Read the model definition and answer for the solid it produces. Units are mm, in the model's axes. A direction names the side the tool comes from. Round coordinates to 2 decimals unless told otherwise and drop trailing zeros. Write each loop counter-clockwise with the first axis right and the second up, starting at its lowest first coordinate (ties: lowest second). Pieces come first, ordered by that corner, then holes. Notation, with made-up numbers: (34, -17.5) - (61, -17.5) arc R29 cw to (61, 21.5) - close; hole circle Ø4 at (35, 57.5). An arc over 180 degrees is marked (long way). One line per item, written item: value. Start each with the question number.
(1) Find the intervals of material crossed by L1, parallel to X at y = 28, z = -6; L2, parallel to X at y = 11, z = -12; L3, parallel to Z at x = -45.5, y = 3, in increasing order.
(2) For faces 4 (the face through (-23, 4, -4)), 5 (the face through (-28.36, 17.04, -6.56)), 6 (the face through (0, 4.8, 0)), 7 (the face through (-35.24, 17.04, -5.67)), determine the directions among +Z, -Z, +X, -X, +Y, -Y from which every point of the face is accessible in a straight line to the end or side of a thin tool.
(3) The mould has two halves that part along Y. Classify faces 1 (the face through (10.2, 15, -3)), 2 (the face through (-25, 0, -4)), 3 (the face through (-31.82, 7.1, -9.68)): +Y half, -Y half, draft (parallel to the pull), parting line (faces both ways), or undercut.
(4) Flat-ended cylindrical pins translate along their axes: pin 1 Ø8 at (x, y) = (-36.5, 24) entering from +Z; pin 2 Ø8 at (x, y) = (-8, 17.5) entering from -Z; pin 3 Ø1.7 at (x, z) = (-54.74, -3.79) entering from +Y; pin 4 Ø4 at (x, y) = (-9.5, 8.5) entering from +Z. Find the tip coordinate at first contact, or state that the pin passes through.
(5) A cutting plane is placed at A-A, the plane y = 5.75. State how many separate pieces and enclosed holes the cut face has, plus the area to 3 significant figures.
(6) A cutting plane is placed at C-C, the plane x = 0. Determine the outline of the cut face in (y, z), plus the area to 3 significant figures.
from build123d import *

# Parameters (mm, degrees)
SKETCH1_W           = 30
SKETCH1_H           = 20
BOSS_EXTRUDE1_DEPTH = 30
SKETCH3_R           = 1.4
SKETCH3_R_2         = 5.2
BOSS_EXTRUDE2_DEPTH = 30
SKETCH2_W           = 20.4
SKETCH2_H           = 20.4
CUT_EXTRUDE1_DEPTH  = 79.115650631
SKETCH9_R           = 7.5
CUT_EXTRUDE5_DEPTH  = 75.606681327
SKETCH5_R           = 8.054275222
SKETCH5_R_2         = 5.25
BOSS_EXTRUDE3_DEPTH = 4
SKETCH7_R           = 2.5
CUT_EXTRUDE3_DEPTH  = 75.606681327
CUT_EXTRUDE4_START  = -10
SKETCH8_R           = 2.5
CUT_EXTRUDE4_DEPTH  = 6
FILLET1_R           = 20
SKETCH10_R          = 2.65
CUT_EXTRUDE6_DEPTH  = 16
FILLET2_R           = 4


with BuildPart() as part:
    # Sketch1 → Boss-Extrude1 (new body)
    with BuildSketch(Plane(origin=(0, 0, 0), x_dir=(1, 0, 0), z_dir=(0, 1, 0))):
        Rectangle(SKETCH1_W, SKETCH1_H)
    extrude(amount=BOSS_EXTRUDE1_DEPTH)

    # Sketch3 → Boss-Extrude2 (add)
    # profile 1 of 2: a face of its own
    with BuildSketch(Plane(origin=(0, 30, 0), x_dir=(1, 0, 0), z_dir=(0, 1, 0))):
        with BuildLine():
            Line((-17.722348511, 16.434098612), (-17.722348511, 9.553228991))
            ThreePointArc((-17.722348511, 9.553228991), (-16.337354231, 9.424239155), (-15, 9.041706549))
            Line((-15, 9.041706549), (-15, 10))
            Line((-15, 10), (15, 10))
            Line((15, 10), (-17.722348511, 16.434098612))
        make_face()
    # profile 2 of 2: a face of its own
    with BuildSketch(Plane(origin=(0, 30, 0), x_dir=(1, 0, 0), z_dir=(0, 1, 0))):
        with BuildLine():
            ThreePointArc((-17.722348511, -5.446771009), (-25.222348511, 2.053228991), (-17.722348511, 9.553228991))
            Line((-17.722348511, 9.553228991), (-17.722348511, 16.434098612))
            Line((-17.722348511, 16.434098612), (-43.266218467, 21.456714216))
            ThreePointArc((-43.266218467, 21.456714216), (-64.731658081, 4.309271536), (-44.280895506, -14.036469069))
            Line((-44.280895506, -14.036469069), (-15, -10))
            Line((-15, -10), (-15, -4.935248568))
            ThreePointArc((-15, -4.935248568), (-16.337354231, -5.317781174), (-17.722348511, -5.446771009))
        make_face()
        with Locations(Location((-46.739009009, -4.205101259, 0), (0, 0, 270))):
            Circle(SKETCH3_R, mode=Mode.SUBTRACT)
        with Locations(Location((-54.739009009, 3.794898741, 0), (0, 0, 270))):
            Circle(SKETCH3_R, mode=Mode.SUBTRACT)
        with Locations(Location((-46.739009009, 3.794898741, 0), (0, 0, 270))):
            Circle(SKETCH3_R_2, mode=Mode.SUBTRACT)
        with Locations(Location((-46.739009009, 11.794898741, 0), (0, 0, 270))):
            Circle(SKETCH3_R, mode=Mode.SUBTRACT)
        with Locations(Location((-38.739009009, 3.794898741, 0), (0, 0, 270))):
            Circle(SKETCH3_R, mode=Mode.SUBTRACT)
    extrude(amount=-BOSS_EXTRUDE2_DEPTH)

    # Sketch2 → Cut-Extrude1 (cut, through all)
    with BuildSketch(Plane.XY.offset(10)):
        with Locations((0, 15)):
            Rectangle(SKETCH2_W, SKETCH2_H)
    extrude(amount=-CUT_EXTRUDE1_DEPTH, mode=Mode.SUBTRACT)

    # Sketch9 → Cut-Extrude5 (cut, through all)
    with BuildSketch(Plane(origin=(0, 30, 0), x_dir=(1, 0, 0), z_dir=(0, 1, 0))):
        with Locations(Location((-17.722348511, 2.053228991, 0), (0, 0, 270))):
            Circle(SKETCH9_R)
    extrude(amount=-CUT_EXTRUDE5_DEPTH, mode=Mode.SUBTRACT)

    # Sketch5 → Boss-Extrude3 (add)
    with BuildSketch(Plane.XZ):
        with Locations((-17.722348511, -2.053228991)):
            Circle(SKETCH5_R)
        with Locations(Location((-17.722348511, -2.053228991, 0), (0, 0, 270))):
            Circle(SKETCH5_R_2, mode=Mode.SUBTRACT)
    extrude(amount=-BOSS_EXTRUDE3_DEPTH)

    # Sketch7 → Cut-Extrude3 (cut, through all)
    with BuildSketch(Plane(origin=(0, 30, 0), x_dir=(1, 0, 0), z_dir=(0, 1, 0))):
        with Locations(Location((0, 2.711092918, 0), (0, 0, 270))):
            Circle(SKETCH7_R)
        with Locations(Location((-32.57112446, 12.062397221, 0), (0, 0, 270))):
            Circle(SKETCH7_R)
    extrude(amount=-CUT_EXTRUDE3_DEPTH, mode=Mode.SUBTRACT)

    # Sketch8 → Cut-Extrude4 (cut)
    # profile 1 of 5: a face of its own
    with BuildSketch(Plane(origin=(0, 30, 0), x_dir=(1, 0, 0), z_dir=(0, 1, 0)).offset(CUT_EXTRUDE4_START)):
        Polygon((-31.673466141, 19.177265611), (-34.093809851, 19.653170637), (-39.980668575, 15.078795072), (-38.888173685, 7.153742712), (-31.478629569, 4.13734486), (-25.161580344, 9.045999369), (-26.254075234, 16.971051729), align=None)
        with Locations(Location((-32.57112446, 12.062397221, 0), (0, 0, 270))):
            Circle(SKETCH8_R, mode=Mode.SUBTRACT)
    # profile 2 of 5: a face of its own
    with BuildSketch(Plane(origin=(0, 30, 0), x_dir=(1, 0, 0), z_dir=(0, 1, 0)).offset(CUT_EXTRUDE4_START)):
        Polygon((-34.093809851, 19.653170637), (-33.66361935, 19.987449581), (-31.673466141, 19.177265611), (-26.415693603, 18.143445347), (-27.334766958, 24.810482895), (-41.061360298, 22.918226238), (-40.792843449, 20.970381801), align=None)
    # profile 3 of 5: a face of its own
    with BuildSketch(Plane(origin=(0, 30, 0), x_dir=(1, 0, 0), z_dir=(0, 1, 0)).offset(CUT_EXTRUDE4_START)):
        Polygon((-26.415693603, 18.143445347), (-31.673466141, 19.177265611), (-26.254075234, 16.971051729), align=None)
    # profile 4 of 5: a face of its own
    with BuildSketch(Plane(origin=(0, 30, 0), x_dir=(1, 0, 0), z_dir=(0, 1, 0)).offset(CUT_EXTRUDE4_START)):
        Polygon((-39.980668575, 15.078795072), (-34.093809851, 19.653170637), (-40.792843449, 20.970381801), align=None)
    # profile 5 of 5: a face of its own
    with BuildSketch(Plane(origin=(0, 30, 0), x_dir=(1, 0, 0), z_dir=(0, 1, 0)).offset(CUT_EXTRUDE4_START)):
        Polygon((-31.673466141, 19.177265611), (-33.66361935, 19.987449581), (-34.093809851, 19.653170637), align=None)
    extrude(amount=-CUT_EXTRUDE4_DEPTH, mode=Mode.SUBTRACT)

    # Fillet1
    fillet1_edges = [part.edges().sort_by_distance(p)[0] for p in [
        (-15, 15, 10),
    ]]
    fillet(fillet1_edges, radius=FILLET1_R)

    # Sketch10 → Cut-Extrude6 (cut)
    with BuildSketch(Plane(origin=(15, 0, 0), x_dir=(0, 0, -1), z_dir=(1, 0, 0))):
        with Locations((0, 15)):
            Circle(SKETCH10_R)
    extrude(amount=-CUT_EXTRUDE6_DEPTH, mode=Mode.SUBTRACT)

    # Fillet2
    fillet2_edges = [part.edges().sort_by_distance(p)[0] for p in [
        (15, 15, 10),
        (15, 15, -10),
    ]]
    fillet(fillet2_edges, radius=FILLET2_R)


solid = part.part
Here are the results:
1. L1: -64.6 to -51.45, -42.03 to -24.1, -11.34 to 15
1. L2: -62.76 to -48.12, -45.35 to -35.07, -30.07 to -10.2
1. L3: -21.75 to -12.45, -11.14 to -8.85, 1.26 to 3.55, 4.86 to 14.16
2. face 4: +Y
2. face 5: none
2. face 6: +Z, -Z
2. face 7: -Z
3. face 1: undercut
3. face 2: -Y half
3. face 3: draft
4. pin 1: z = 13.52
4. pin 2: z = -15.31
4. pin 3: through
4. pin 4: z = 10
5. separate pieces: 2
5. enclosed holes: 7
5. area: 1,410 mm²
6. outline: (0, -12.95) - (4.8, -12.95) - (4.8, -5.21) - (0, -5.21) - close; (0, -0.21) - (4.8, -0.21) - (4.8, 10) - (0, 10) - close; (25.2, -12.95) - (30, -12.95) - (30, -5.21) - (25.2, -5.21) - close; (25.2, -0.21) - (30, -0.21) - (30, 10) - (25.2, 10) - close
6. area: 172 mm²
